Autodesk Inventor part; units mm, degrees
ref_plane "YZ Plane" through (0, 0, 0) normal (1, 0, 0) x (0, 1, 0)
ref_plane "XZ Plane" through (0, 0, 0) normal (0, 1, 0) x (-1, 0, 0)
ref_plane "XY Plane" through (0, 0, 0) normal (0, 0, 1) x (1, 0, 0)
sketch "Sketch1" plane through (0, 0, 0) normal (0, 0, 1) x (1, 0, 0)
  point P0 (0, 0)
sketch "Sketch2" plane through (0, 0, 0) normal (0, 0, 1) x (1, 0, 0)
  line L0 (-58, -60) -> (-60, -60)
  line L1 (-60, -60) -> (-60, -39.5)
  line L2 (-60, -39.5) -> (-58, -39.5)
  line L3 (-58, -39.5) -> (-58, -60)
  line L4 (49.6, 30) -> (51.6, 30)
  line L5 (51.6, 30) -> (51.6, 9.5)
  line L6 (51.6, 9.5) -> (49.6, 9.5)
  line L7 (49.6, 9.5) -> (49.6, 30)
  line L8 (-58, 39.5) -> (-60, 39.5)
  line L9 (-60, 39.5) -> (-60, 60)
  line L10 (-60, 60) -> (-58, 60)
  line L11 (-58, 60) -> (-58, 39.5)
  line L12 (-21.6, -39.5) -> (-19.6, -39.5)
  line L13 (-19.6, -39.5) -> (-19.6, -60)
  line L14 (-19.6, -60) -> (-21.6, -60)
  line L15 (-21.6, -60) -> (-21.6, -39.5)
  line L16 (51.6, -30) -> (49.6, -30)
  line L17 (49.6, -30) -> (49.6, -9.5)
  line L18 (49.6, -9.5) -> (51.6, -9.5)
  line L19 (51.6, -9.5) -> (51.6, -30)
  line L20 (-21.6, 60) -> (-19.6, 60)
  line L21 (-19.6, 60) -> (-19.6, 39.5)
  line L22 (-19.6, 39.5) -> (-21.6, 39.5)
  line L23 (-21.6, 39.5) -> (-21.6, 60)
  line L24 (90, -35) -> (90, 35)
  line L25 (90, 35) -> (49.6, 35)
  line L26 (49.6, 35) -> (49.6, 60)
  line L27 (49.6, 60) -> (90, 60)
  line L28 (90, 60) -> (90, 90)
  line L29 (90, 90) -> (-19.6, 90)
  line L30 (-19.6, 90) -> (-19.6, 65)
  line L31 (-19.6, 65) -> (-60, 65)
  line L32 (-60, 65) -> (-60, 90)
  line L33 (-60, 90) -> (-90, 90)
  line L34 (-90, 90) -> (-90, -90)
  line L35 (-90, -90) -> (-60, -90)
  line L36 (-60, -90) -> (-60, -65)
  line L37 (-60, -65) -> (-19.6, -65)
  line L38 (-19.6, -65) -> (-19.6, -90)
  line L39 (-19.6, -90) -> (90, -90)
  line L40 (90, -90) -> (90, -60)
  line L41 (90, -60) -> (49.6, -60)
  line L42 (49.6, -60) -> (49.6, -35)
  line L43 (49.6, -35) -> (90, -35)
  line L44 (86, -32) -> (73.8, -32)
  line L45 (73.8, -32) -> (73.8, -7.5)
  line L46 (73.8, -7.5) -> (86, -7.5)
  line L47 (86, -7.5) -> (86, -32)
  line L48 (65.8, -32) -> (53.6, -32)
  line L49 (53.6, -32) -> (53.6, -7.5)
  line L50 (53.6, -7.5) -> (65.8, -7.5)
  line L51 (65.8, -7.5) -> (65.8, -32)
  line L52 (86, -86) -> (70.6, -86)
  line L53 (70.6, -86) -> (70.6, -69.8)
  line L54 (70.6, -69.8) -> (86, -69.8)
  line L55 (86, -69.8) -> (86, -86)
  line L56 (86, 86) -> (86, 69.8)
  line L57 (86, 69.8) -> (70.6, 69.8)
  line L58 (70.6, 69.8) -> (70.6, 86)
  line L59 (70.6, 86) -> (86, 86)
  line L60 (73.8, 32) -> (86, 32)
  line L61 (86, 32) -> (86, 7.5)
  line L62 (86, 7.5) -> (73.8, 7.5)
  line L63 (73.8, 7.5) -> (73.8, 32)
  line L64 (65.8, 32) -> (65.8, 7.5)
  line L65 (65.8, 7.5) -> (53.6, 7.5)
  line L66 (53.6, 7.5) -> (53.6, 32)
  line L67 (53.6, 32) -> (65.8, 32)
  line L68 (-69.6, -87) -> (-85, -87)
  line L69 (-85, -87) -> (-85, -70.8)
  line L70 (-85, -70.8) -> (-69.6, -70.8)
  line L71 (-69.6, -70.8) -> (-69.6, -87)
  line L72 (-56, -62) -> (-56, -37.5)
  line L73 (-56, -37.5) -> (-43.8, -37.5)
  line L74 (-43.8, -37.5) -> (-43.8, -62)
  line L75 (-43.8, -62) -> (-56, -62)
  line L76 (-56, 62) -> (-43.8, 62)
  line L77 (-43.8, 62) -> (-43.8, 37.5)
  line L78 (-43.8, 37.5) -> (-56, 37.5)
  line L79 (-56, 37.5) -> (-56, 62)
  line L80 (-23.6, 62) -> (-23.6, 37.5)
  line L81 (-23.6, 37.5) -> (-35.8, 37.5)
  line L82 (-35.8, 37.5) -> (-35.8, 62)
  line L83 (-35.8, 62) -> (-23.6, 62)
  line L84 (-23.6, -62) -> (-35.8, -62)
  line L85 (-35.8, -62) -> (-35.8, -37.5)
  line L86 (-35.8, -37.5) -> (-23.6, -37.5)
  line L87 (-23.6, -37.5) -> (-23.6, -62)
  line L88 (-85, 87) -> (-69.6, 87)
  line L89 (-69.6, 87) -> (-69.6, 70.8)
  line L90 (-69.6, 70.8) -> (-85, 70.8)
  line L91 (-85, 70.8) -> (-85, 87)
  line L92 (46.6, 35) -> (49.6, 35)
  line L93 (49.6, 35) -> (49.6, 60)
  line L94 (49.6, 60) -> (84, 60)
  line L95 (84, 63) -> (43.6, 63)
  line L96 (46.6, 57) -> (46.6, 35)
  line L97 (90, 90) -> (87, 90)
  line L98 (87, 90) -> (87, 63)
  line L99 (87, 63) -> (90, 63)
  line L100 (90, 63) -> (90, 90)
  line L101 (87, 90) -> (-19.6, 90)
  line L102 (-19.6, 90) -> (-19.6, 87)
  line L103 (-19.6, 87) -> (87, 87)
  line L104 (87, 87) -> (87, 90)
  line L105 (-19.6, 90) -> (-16.6, 90)
  line L106 (-16.6, 90) -> (-16.6, 65)
  line L107 (-16.6, 65) -> (-19.6, 65)
  line L108 (-19.6, 65) -> (-19.6, 90)
  line L109 (-19.6, 90) -> (-13.6, 90)
  line L110 (-13.6, 90) -> (-13.6, 84)
  line L111 (-13.6, 84) -> (-19.6, 84)
  line L112 (-19.6, 84) -> (-19.6, 90)
  line L113 (90, 60) -> (84, 60)
  line L114 (84, 60) -> (84, 66)
  line L115 (84, 66) -> (90, 66)
  line L116 (90, 66) -> (90, 60)
  line L117 (-19.6, 65) -> (-16.6, 65)
  line L118 (-16.6, 65) -> (-16.6, 68)
  line L119 (-16.6, 68) -> (-19.6, 68)
  line L120 (-19.6, 68) -> (-19.6, 65)
  line L121 (-19.6, 68) -> (-13.6, 68)
  line L122 (-13.6, 68) -> (-13.6, 62)
  line L123 (-13.6, 62) -> (-19.6, 62)
  line L124 (-19.6, 62) -> (-19.6, 68)
  line L125 (46.6, 90) -> (52.6, 90)
  line L126 (52.6, 90) -> (52.6, 84)
  line L127 (52.6, 84) -> (46.6, 84)
  line L128 (46.6, 84) -> (46.6, 90)
  line L129 (84, 60) -> (84, 63)
  circle A0 centre (-63, -65) radius 1.5
  circle A1 centre (-16.6, -87) radius 1.5
  circle A2 centre (49.6, -87) radius 1.5
  circle A3 centre (46.6, -60) radius 1.5
  circle A4 centre (87, -63) radius 1.5
  circle A5 centre (46.6, -32) radius 1.5
  circle A6 centre (46.6, 32) radius 1.5
  circle A7 centre (87, 63) radius 1.5
  circle A8 centre (46.6, 60) radius 1.5
  circle A9 centre (49.6, 87) radius 1.5
  circle A10 centre (-16.6, 87) radius 1.5
  circle A11 centre (-16.6, 65) radius 1.5
  circle A12 centre (-63, 65) radius 1.5
  line L130 (43.6, 63) -> (43.6, 57)
  line L131 (43.6, 57) -> (46.6, 57)
  point P0 (0, 0)
  point P1 (90, 63)
  point P2 (87, 66)
  point P3 (-16.6, 84)
  point P4 (-13.6, 87)
  point P5 (46.6, 87)
  point P6 (52.6, 87)
  dimension "d0" = 3
  dimension "d1" = 3
  dimension "d2" = 6
  dimension "d3" = 6
  dimension "d4" = 6
  dimension "d5" = 6
  dimension "d6" = 3
  dimension "d7" = 6
  dimension "d8" = 6
extrude "Extrusion1" add sketch "Sketch2" along normal blind 8 contours L114 L115 L98 A7 L99 L28 L27 | L99 A7 L98 L115 L28 | L115 L98 L29 L28 | A7 L98 L99 | L99 L98 A7 | L103 L126 L29 L98 | L126 L127 L128 L103 A9 | L103 A9 L128 L29 L126 | A9 L103 | L103 A9 | L128 L103 L110 L29 | L110 L103 A10 L106 L29 | L106 A10 L103 L30 L29 | L110 L111 L106 A10 L103 | L30 L119 L106 A11 L107 | L107 A11 L106 L121 L122 L123 L124 | A10 L103 L106 | L106 L103 A10 | A10 L106 L103 | L30 L111 L106 L119 | A11 L106 L107 | L107 L106 A11 | L103 A10 L106 L111 L30 | L106 A10 L103
sketch "Sketch3" plane through (0, 0, 0) normal (0, 0, -1) x (-1, 0, 0)
  line L0 (-87, 66) -> (-84, 66)
  line L1 (-84, 60) -> (-90, 60)
  line L2 (-84, 66) -> (-90, 66)
  line L3 (-90, 66) -> (-90, 60)
  line L4 (-90, 60) -> (-84, 60)
  line L5 (-84, 60) -> (-84, 66)
  point P0 (0, 0)
extrude "Extrusion2" cut sketch "Sketch3" against normal blind 3
sketch "Sketch4" plane through (0, 0, 3) normal (0, 0, -1) x (-1, 0, 0)
  line L0 (-87, 66) -> (-84, 66)
  line L1 (-90, 60) -> (-90, 90)
  line L2 (-84, 66) -> (-90, 60)
  line L3 (-90, 60) -> (-90, 66)
  line L4 (-84, 66) -> (-84, 60)
  line L5 (-90, 66) -> (-84, 60)
  circle A0 centre (-87, 63) radius 2
  point P0 (0, 0)
  dimension "d13" = 4
extrude "Extrusion3" cut sketch "Sketch4" against normal blind 4 contours A0 L5 L2 | L2 L5 A0 | A0 L2 L5 | L2 A0 L5
sketch "Sketch5" plane through (0, 0, 8) normal (0, 0, 1) x (1, 0, 0)
  line L0 (-13.6, 62) -> (-13.6, 68)
  line L1 (-19.6, 62) -> (-13.6, 62)
  line L2 (-13.6, 68) -> (-19.6, 68)
  line L3 (-19.6, 68) -> (-19.6, 62)
  line L4 (-19.6, 62) -> (-13.6, 62)
  line L5 (-13.6, 62) -> (-13.6, 68)
  point P0 (0, 0)
extrude "Extrusion4" cut sketch "Sketch5" against normal blind 5
sketch "Sketch6" plane through (0, 0, 3) normal (0, 0, 1) x (1, 0, 0)
  line L0 (-13.6, 68) -> (-13.6, 62)
  line L1 (-19.6, 62) -> (-19.6, 68)
  line L2 (-13.6, 68) -> (-19.6, 62)
  line L3 (-19.6, 62) -> (-19.6, 68)
  line L4 (-19.6, 68) -> (-13.6, 62)
  circle A0 centre (-16.6, 65) radius 1.65
  point P0 (0, 0)
  dimension "d18" = 3.3
extrude "Extrusion5" cut sketch "Sketch6" against normal blind 3 contours A0 L4 L2 | L2 L4 A0 | A0 L2 L4 | L2 A0 L4
sketch "Sketch7" plane through (0, 0, 0) normal (0, 0, -1) x (-1, 0, 0)
  point P0 (0, 0)
sketch "Sketch8" plane through (0, 0, 0) normal (0, 0, -1) x (-1, 0, 0)
  line L0 (-46.6, 84) -> (-52.6, 84)
  line L1 (-90, 90) -> (19.6, 90)
  line L2 (-52.6, 84) -> (-46.6, 84)
  line L3 (-46.6, 84) -> (-46.6, 90)
  line L4 (-46.6, 90) -> (-52.6, 90)
  line L5 (-52.6, 90) -> (-52.6, 84)
  line L6 (-52.6, 84) -> (-46.6, 90)
  line L7 (-46.6, 84) -> (-52.6, 90)
  circle A0 centre (-49.6, 87) radius 2
  line L8 (19.6, 90) -> (13.6, 90)
  line L9 (13.6, 90) -> (13.6, 84)
  line L10 (13.6, 84) -> (19.6, 84)
  line L11 (19.6, 84) -> (19.6, 90)
  line L12 (19.6, 90) -> (13.6, 84) construction
  line L13 (13.6, 90) -> (19.6, 84) construction
  line L14 (13.6, 84) -> (13.6, 87)
  circle A1 centre (16.6, 87) radius 2
  point P0 (0, 0)
  dimension "d21" = 6
  dimension "d22" = 4
  dimension "d23" = 6
  dimension "d24" = 6
  dimension "d25" = 4
extrude "Extrusion6" cut sketch "Sketch8" against normal blind 6 contours A0 L6 L7 | L7 L6 A0 | A0 L7 L6 | L6 L7 A0 | A1
fillet "Fillet1" radius 3 4 edges at (-13.6, 62, 1.5) (-13.6, 68, 1.5) (46.6, 84, 4) (52.6, 84, 4)
fillet "Fillet2" radius 3 1 edges at (-13.6, 84, 4)
fillet "Fillet3" radius 3 1 edges at (84, 66, 5.5)
properties part number "leftwall2"
Could you check a few things on this model? Use its own coordinates, in mm. A direction names the side the tool comes from. Round coordinates to 2 decimals unless told otherwise and drop trailing zeros. Write each loop counter-clockwise with the first axis right and the second up, starting at its lowest first coordinate (ties: lowest second). Pieces come first, ordered by that corner, then holes. Notation, with made-up numbers: (64.25, 78) - (106.25, 78) arc R5 cw to (106.25, 87) - close; hole circle Ø1 at (-34, 58.5). An arc over 180 degrees is marked (long way). Use a Markdown table: item, result.
Q1. For pin 1 (2 mm diameter, centred on x = 86.5, y = 63, fed in from -Z); pin 2 (3 mm diameter, centred on x = 86.5, y = 61.5, fed in from -Z); pin 3 (1.5 mm diameter, centred on x = -18.5, z = 2, fed in from -Y), each with a flat end and sliding along its axis, tell me the tip position at first contact or that it passes through.
Output values:
| item | result |
|---|---|
| pin 1 | z = 7 |
| pin 2 | z = 3 |
| pin 3 | y = 62 |
Q2. For faces 1 (the cylindrical face through (47.46, 84.9, 4.06)), 2 (the flat face through (-18, 68, 6)), 3 (the flat face through (88, 66, 1)), 4 (the flat face through (-16.6, 76, 4)), 5 (the cylindrical face through (-16.34, 88.983, 2.958)), which set-ups out of +Z, -Z, +X, -X, +Y, -Y let a thin tool reach every point of the face, with its end or its side?
Output values:
| item | result |
|---|---|
| face 1 | +Z, -Z, -Y |
| face 2 | +Z, -X, -Y |
| face 3 | -Z, +X, -Y |
| face 4 | +Z, -Z |
| face 5 | -Z |
Q3. I want a section at C-C (x = 13). List the corners of the cut face in (y, z) for me, plus the area to 3 significant figures.
Output values:
| item | result |
|---|---|
| outline | (87, 0) - (90, 0) - (90, 8) - (87, 8) - close |
| area | 24.0 mm2 |
Q4. I want a section at B-B (z = 2). Count the separate pieces of the cut face and the enclosed holes in it, plus the area to 3 significant figures.
Output values:
| item | result |
|---|---|
| separate pieces | 1 |
| enclosed holes | 3 |
| area | 468 mm2 |
Q5. I want a section at A-A (y = 77.75). List the corners of the cut face in (x, z) for me, plus the area to 3 significant figures.
Output values:
| item | result |
|---|---|
| outline | (-19.6, 0) - (-16.6, 0) - (-16.6, 8) - (-19.6, 8) - close; (87, 0) - (90, 0) - (90, 8) - (87, 8) - close |
| area | 48.0 mm2 |
Q6. Please list where these lines run through material, in increasing order: L1, parallel to X at y = 73.5, z = 2; L2, parallel to X at y = 65.25, z = 1.5; L3, parallel to Y at x = 49.6, z = 4.1.
Output values:
| item | result |
|---|---|
| L1 | -19.6 to -16.6, 87 to 90 |
| L2 | -19.6 to -18.23, -14.97 to -13.61 |
| L3 | 84 to 85, 89 to 90 |
Q7. Thinking about a two-plate mould opening in X: for faces 6 (the cylindrical face through (-14.46, 67.1, 1.52)), 7 (the flat face through (-18, 62, 1)), 8 (the cylindrical face through (49.86, 88.983, 2.958)), 9 (the cylindrical face through (-14.5, 62.86, 1.52)), which applies, released by +X, released by -X, zero draft, split by the parting line, or undercut?
Output values:
| item | result |
|---|---|
| face 6 | undercut |
| face 7 | zero draft |
| face 8 | undercut |
| face 9 | released by +X |
